The model under review builds one solid part; all positions refer to its coordinate system, in mm. Give positions to 0.01 mm unless a question says otherwise; leave off trailing zeros. Order: outer loops, then holes, each group sorted by start corner. A loop starts at its lowest first (then second) coordinate and runs counter-clockwise, first axis right, second up. Notation, with made-up numbers: (32.5, -11.5) -> (38.5, -11.5) arc R18 ccw to (38.5, -3.5) -> close; hole circle Ø7 at (-23.5, 49). An arc over 180 degrees is marked (long way). Use one line per item in the form item = value.
```python
from build123d import *

# Parameters (mm, degrees)
MODEL_R         = 0.65
MODEL_R_2       = 3.4746057
EXTRUDE_1_DEPTH = 0.5
EXTRUDE1_START  = -0.5
EXTRUDE1_DEPTH  = 1
EXTRUDE2_START  = -0.1
EXTRUDE2_DEPTH  = 0.1


# Read off the part's stored shape, not the designer's step: Extrude1
with BuildPart() as part:
    # Model → Бобышка-Вытянуть1 (new, symmetric)
    with BuildSketch(Plane.XY):
        with BuildLine():
            Line((0.65, -4.7), (0.65, -5.5))
            Line((0.65, -5.5), (12.5, -5.5))
            Line((12.5, -5.5), (12.5, 5.5))
            Line((12.5, 5.5), (0.65, 5.5))
            Line((0.65, 5.5), (0.65, 4.7))
            ThreePointArc((0.65, 4.7), (0, 4.05), (-0.65, 4.7))
            Line((-0.65, 4.7), (-0.65, 5.5))
            Line((-0.65, 5.5), (-10, 5.5))
            Line((-10, 5.5), (-10, -5.5))
            Line((-10, -5.5), (-0.65, -5.5))
            Line((-0.65, -5.5), (-0.65, -4.7))
            ThreePointArc((-0.65, -4.7), (0, -4.05), (0.65, -4.7))
        make_face()
        with Locations((-8.5, 0)):
            Circle(MODEL_R, mode=Mode.SUBTRACT)
        Circle(MODEL_R_2, mode=Mode.SUBTRACT)
        with Locations((11, 0)):
            Circle(MODEL_R, mode=Mode.SUBTRACT)
    extrude(amount=EXTRUDE_1_DEPTH, both=True)

    # Extrude1 outline → Extrude1 (cut)
    with BuildSketch(Plane.XY.offset(EXTRUDE1_START)):
        with BuildLine():
            ThreePointArc((11.22497216, 5.5), (12.177071733, 2.822928267), (12.5, 0))
            Line((12.5, 0), (12.5, 5.5))
            Line((12.5, 5.5), (11.22497216, 5.5))
        make_face()
        with BuildLine():
            ThreePointArc((12.5, 0), (12.177071733, -2.822928267), (11.22497216, -5.5))
            Line((11.22497216, -5.5), (12.5, -5.5))
            Line((12.5, -5.5), (12.5, 0))
        make_face()
        with BuildLine():
            ThreePointArc((-8.351646544, -5.5), (-9.579051769, -2.87084782), (-10, 2.7e-08))
            Line((-10, 2.7e-08), (-10, -5.5))
            Line((-10, -5.5), (-8.351646544, -5.5))
        make_face()
        with BuildLine():
            ThreePointArc((-10, 2.7e-08), (-9.579051761, 2.870847846), (-8.351646544, 5.5))
            Line((-8.351646544, 5.5), (-10, 5.5))
            Line((-10, 5.5), (-10, 2.7e-08))
        make_face()
    extrude(amount=EXTRUDE1_DEPTH, mode=Mode.SUBTRACT)

    # Sketch2 → Extrude2 (cut)
    # profile 1 of 3: a face of its own
    with BuildSketch(Plane.XY.offset(0.5).offset(EXTRUDE2_START)):
        with BuildLine():
            Line((-5.6, -5.5), (-5.1, -5.5))
            Line((-5.1, -5.5), (-5.1, -2))
            Line((-5.1, -2), (-3.7, -2))
            Line((-3.7, -2), (-2.841282241, -2))
            ThreePointArc((-2.841282241, -2), (-2.969532083, -1.804096444), (-3.084296479, -1.6))
            Line((-3.084296479, -1.6), (-4.1, -1.6))
            Line((-4.1, -1.6), (-5.6, -1.6))
            Line((-5.6, -1.6), (-5.6, -5.5))
        make_face()
    # profile 2 of 3: a face of its own
    with BuildSketch(Plane.XY.offset(0.5).offset(EXTRUDE2_START)):
        with BuildLine():
            Line((-7.5, -5.5), (-7.1, -5.5))
            Line((-7.1, -5.5), (-7.1, -1.6))
            Line((-7.1, -1.6), (-7.1, 1.6))
            Line((-7.1, 1.6), (-4.1, 1.6))
            Line((-4.1, 1.6), (-3.084296479, 1.6))
            ThreePointArc((-3.084296479, 1.6), (-2.969532083, 1.804096444), (-2.841282241, 2))
            Line((-2.841282241, 2), (-3.7, 2))
            Line((-3.7, 2), (-7.5, 2))
            Line((-7.5, 2), (-7.5, -2))
            Line((-7.5, -2), (-7.5, -5.5))
        make_face()
    # profile 3 of 3: a face of its own
    with BuildSketch(Plane.XY.offset(0.5).offset(EXTRUDE2_START)):
        with BuildLine():
            Line((4.6, -4.5), (11.66190379, -4.5))
            ThreePointArc((11.66190379, -4.5), (11.754970287, -4.250961487), (11.842719282, -4))
            Line((11.842719282, -4), (9.1, -4))
            Line((9.1, -4), (5.1, -4))
            Line((5.1, -4), (5.1, -1.5))
            Line((5.1, -1.5), (6.1, -1.5))
            Line((6.1, -1.5), (9.1, -1.5))
            Line((9.1, -1.5), (9.1, -2.5))
            Line((9.1, -2.5), (12.247448714, -2.5))
            ThreePointArc((12.247448714, -2.5), (12.295747488, -2.250465219), (12.338962679, -2))
            Line((12.338962679, -2), (9.6, -2))
            Line((9.6, -2), (9.6, -1.5))
            Line((9.6, -1.5), (9.6, 1.5))
            Line((9.6, 1.5), (9.6, 2))
            Line((9.6, 2), (12.338962679, 2))
            ThreePointArc((12.338962679, 2), (12.295747488, 2.250465219), (12.247448714, 2.5))
            Line((12.247448714, 2.5), (9.1, 2.5))
            Line((9.1, 2.5), (9.1, 1.5))
            Line((9.1, 1.5), (6.1, 1.5))
            Line((6.1, 1.5), (5.1, 1.5))
            Line((5.1, 1.5), (5.1, 4))
            Line((5.1, 4), (9.1, 4))
            Line((9.1, 4), (11.842719282, 4))
            ThreePointArc((11.842719282, 4), (11.754970287, 4.250961487), (11.66190379, 4.5))
            Line((11.66190379, 4.5), (4.6, 4.5))
            Line((4.6, 4.5), (4.6, 4))
            Line((4.6, 4), (4.6, 1.5))
            Line((4.6, 1.5), (4.6, -1.5))
            Line((4.6, -1.5), (4.6, -4))
            Line((4.6, -4), (4.6, -4.5))
        make_face()
        Polygon((9.1, 1), (9.1, -1), (6.1, -1), (5.1, -1), (5.1, 0.813952094), (5.1, 1), (6.1, 1), align=None, mode=Mode.SUBTRACT)
    extrude(amount=EXTRUDE2_DEPTH, mode=Mode.SUBTRACT)


solid = part.part
```
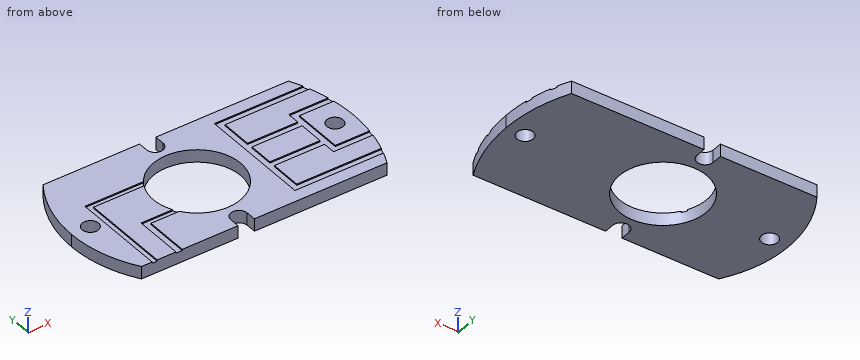
1. Add section B-B on x = 7.75. Give the boundary of the cut face in (y, z).
Values:
outline = (-5.5, -0.5) -> (5.5, -0.5) -> (5.5, 0.5) -> (4.5, 0.5) -> (4.5, 0.4) -> (4, 0.4) -> (4, 0.5) -> (1.5, 0.5) -> (1.5, 0.4) -> (1, 0.4) -> (1, 0.5) -> (-1, 0.5) -> (-1, 0.4) -> (-1.5, 0.4) -> (-1.5, 0.5) -> (-4, 0.5) -> (-4, 0.4) -> (-4.5, 0.4) -> (-4.5, 0.5) -> (-5.5, 0.5) -> close
2. For L1, parallel to Y at x = 7.75, z = 0.45; L2, parallel to Y at x = 11, z = 0.05; L3, parallel to Y at x = 0, z = 0.15, list the stretches that pass through material, from the lowest coordinate up.
Values:
L1 = -5.5 to -4.5, -4 to -1.5, -1 to 1, 1.5 to 4, 4.5 to 5.5
L2 = -5.5 to -0.65, 0.65 to 5.5
L3 = -4.05 to -3.47, 3.47 to 4.05
3. Add section A-A on x = 0. Give the boundary of the cut face in (y, z).
Values:
outline = (-4.05, -0.5) -> (-3.47, -0.5) -> (-3.47, 0.5) -> (-4.05, 0.5) -> close; (3.47, -0.5) -> (4.05, -0.5) -> (4.05, 0.5) -> (3.47, 0.5) -> close
4. Add section C-C on z = -0.2. Give the boundary of the cut face in (x, y), then the cut area to 3 significant figures.
Values:
outline = (-8.35, -5.5) -> (-0.65, -5.5) -> (-0.65, -4.7) arc R0.65 cw to (0.65, -4.7) -> (0.65, -5.5) -> (11.22, -5.5) arc R12.5 ccw to (11.22, 5.5) -> (0.65, 5.5) -> (0.65, 4.7) arc R0.65 cw to (-0.65, 4.7) -> (-0.65, 5.5) -> (-8.35, 5.5) arc R10 ccw to start; hole circle Ø1.3 at (-8.5, 0); hole circle Ø6.95 at (0, 0); hole circle Ø1.3 at (11, 0)
area = 193 mm^2
5. Add section D-D on y = -5. Give the boundary of the cut face in (x, z).
Values:
outline = (-8.66, -0.5) -> (-0.65, -0.5) -> (-0.65, 0.5) -> (-5.1, 0.5) -> (-5.1, 0.4) -> (-5.6, 0.4) -> (-5.6, 0.5) -> (-7.1, 0.5) -> (-7.1, 0.4) -> (-7.5, 0.4) -> (-7.5, 0.5) -> (-8.66, 0.5) -> close; (0.65, -0.5) -> (11.46, -0.5) -> (11.46, 0.5) -> (0.65, 0.5) -> close
